Autodesk Inventor part; units mm, degrees
ref_plane "YZ Plane" through (0, 0, 0) normal (1, 0, 0) x (0, 1, 0)
ref_plane "XZ Plane" through (0, 0, 0) normal (0, 1, 0) x (-1, 0, 0)
ref_plane "XY Plane" through (0, 0, 0) normal (0, 0, 1) x (1, 0, 0)
sketch "Sketch1" plane through (0, 0, 0) normal (0, 0, 1) x (1, 0, 0)
  line L0 (-3.8891, 0) -> (0, -3.8891)
  line L1 (0, -3.8891) -> (3.8891, 0)
  line L2 (3.8891, 0) -> (0, 3.8891)
  line L3 (0, 3.8891) -> (-3.8891, 0)
  line L4 (-3.8891, 0) -> (3.8891, 0) construction
  line L5 (0, -3.8891) -> (0, 3.8891) construction
  point P0 (0, 0)
  dimension "d0" = 5.5
  dimension "d1" = 5.5
  dimension "d2" = 90
  dimension "d3" = 5.5
  dimension "d4" = 90
  dimension "d5" = 0
  dimension "d6" = 0
extrude "Extrusion1" add sketch "Sketch1" along normal blind 3
sketch "Sketch2" plane through (0, 0, 0) normal (1, 0, 0) x (0, 1, 0)
  line L0 (3.8891, 0) -> (0, 0)
  line L1 (3.8891, 0) -> (3.8891, 0.75)
  line L2 (3.8891, 0.75) -> (3.1391, 0)
  line L3 (3.8891, 0) -> (3.1391, 0)
  line L4 (-3.8891, 3) -> (0, 3)
  line L5 (0, 3) -> (0, 0)
  dimension "d9" = 0.75
  dimension "d10" = 0.75
revolve "Revolution1" cut sketch "Sketch2" angle 360 about axis through (0, 0, 3) along (0, 0, -1)
sketch "Sketch3" plane through (0, 0, 3) normal (0, 0, 1) x (1, 0, 0)
  circle A0 centre (0, 0) radius 2.1
  dimension "d12" = 4.2
extrude "Extrusion2" add sketch "Sketch3" along normal blind 55.206
chamfer "Chamfer1" distance 1 angle 45 1 edges at (-2.1, 0, 58.206)
thread "Thread1"
properties part number "ES117_Bolt" material "Stainless Steel"
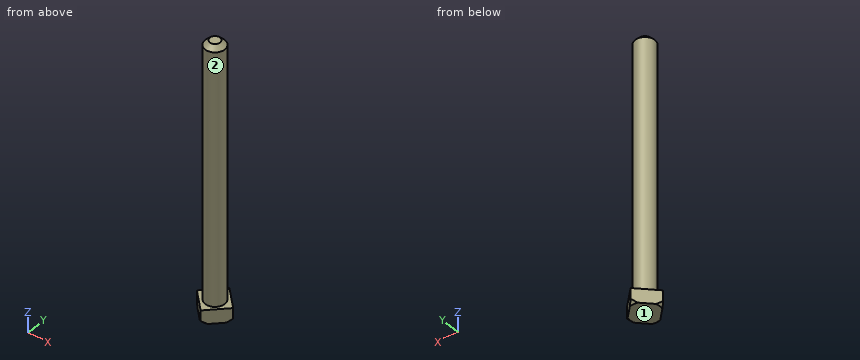
Read the model definition and answer for the solid it produces. Units are mm, in the model's axes. Face numbers are marked on the shaded views. A direction names the side the tool comes from. Round coordinates to 2 decimals unless told otherwise and drop trailing zeros. Loops run counter-clockwise (first coordinate to the right, second up) from the corner with the lowest first, then second, coordinate; pieces in that order, holes last.
Q1. Consider probe 1 along Z at (x, y) = (0, -2.5); probe 2 along X at (y, z) = (-1, 18); probe 3 along Z at (x, y) = (0.5, -1.75). Determine where each line is inside the solid, lowest interval first.
Q2. Which of the six approach directions +Z, -Z, +X, -X, +Y, -Y give full straight-line access (tool end or side, diameter ignored) to the marked faces 1 and 2?
Q3. Each of these flat-tipped pins is pushed along its axis until it touches: pin 1 (1.5 mm diameter, centred on x = -1, z = 52, fed in from +Y); pin 2 (3 mm diameter, centred on y = 1, z = 8, fed in from +X). Where does it stop, or does it pass through?
Q4. Section A-A on z = 30.5 is taken. Write down the section's boundary in (x, y).
Output:
1. probe 1: z = 0 to 3
1. probe 2: x = -1.85 to 1.85
1. probe 3: z = 0 to 57.49
2. face 1: -Z, +X, -X, +Y, -Y
2. face 2: +Z
3. pin 1: stops at y = 2.09
3. pin 2: stops at x = 2.1
4. outline: circle Ø4.2 at (0, 0)
